from build123d import *

# Parameters (mm, degrees)
SKETCH1_R           = 13
BOSS_EXTRUDE1_DEPTH = 25
SKETCH2_R           = 4
CUT_EXTRUDE1_DEPTH  = 8
SKETCH4_W           = 4.368412871
SKETCH4_H           = 18.958156908


with BuildPart() as part:
    # Sketch1 → Boss-Extrude1 (new body)
    with BuildSketch(Plane(origin=(0, 0, 0), x_dir=(1, 0, 0), z_dir=(0, 1, 0))):
        with Locations(Location((0, 0, 0), (0, 0, 270))):
            Circle(SKETCH1_R)
    extrude(amount=BOSS_EXTRUDE1_DEPTH)

    # Sketch2 → Cut-Extrude1 (cut)
    with BuildSketch(Plane(origin=(0, 25, 0), x_dir=(1, 0, 0), z_dir=(0, 1, 0))):
        with Locations(Location((0, 0, 0), (0, 0, 270))):
            Circle(SKETCH2_R)
    extrude(amount=-CUT_EXTRUDE1_DEPTH, mode=Mode.SUBTRACT)

    # Sketch4 → Cut-Revolve1 (revolve, cut)
    with BuildSketch(Plane.XY, mode=Mode.PRIVATE) as cut_revolve1_sk:
        with BuildLine():
            ThreePointArc((0, 0), (-9.192388155, 3.807611845), (-13, 13))
            Line((-13, 13), (-13, -5.958156908))
            Line((-13, -5.958156908), (0, -5.958156908))
            Line((0, -5.958156908), (0, 0))
        make_face()
        with Locations((-15.184206436, 3.520921546)):
            Rectangle(SKETCH4_W, SKETCH4_H)
    revolve(cut_revolve1_sk.sketch.rotate(Axis((0, -5.958156908, 0), (0, 1, 0)), 270), axis=Axis((0, -5.958156908, 0), (0, 1, 0)), mode=Mode.SUBTRACT)


solid = part.part
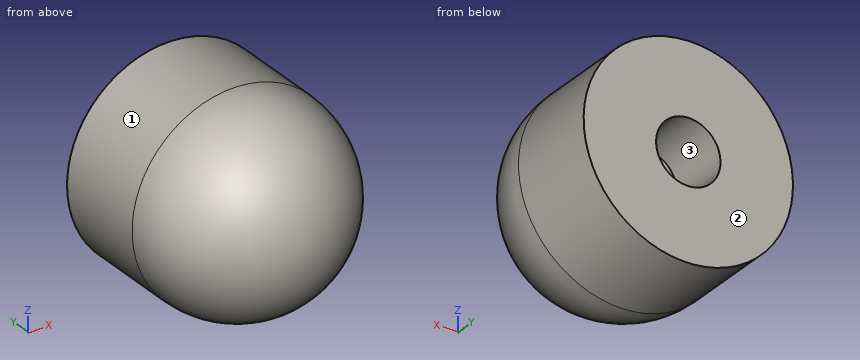
Source: CAD feature listing. Evaluate the final solid. Frame: model axes, mm. Face numbers are marked on the shaded views. Round coordinates to 2 decimals unless told otherwise and drop trailing zeros. Loops run counter-clockwise (first coordinate to the right, second up) from the corner with the lowest first, then second, coordinate; pieces in that order, holes last.
Q1. Section A-A, the plane y = 19.75. Return loops of the section in (x, z), plus the area to 3 significant figures.
Q2. Section B-B, the plane x = 0. Return loops of the section in (y, z).
Q3. Mould query, pull axis X, two halves, no side actions, for the marked faces 1, 2 and 3. Classes: pulls with the +X half, pulls with the -X half, needs draft (parallel to the pull), parting line crosses it, or undercut.
Q4. Section C-C, the plane z = 0. Return loops of the section in (x, y).
Q5. Section D-D, the plane y = 11. Return loops of the section in (x, z).
Q6. Ray query, line 1 (X direction, y = 22.5, z = 0); line 2 (Z direction, x = -5.25, y = 14); line 3 (X direction, y = 6.5, z = 4.5). Return the intervals inside material, ascending.
Q7. First-contact query: P1, Ø8, axis at x = -6.5, y = 17.5, coming from the +Z side; P2, Ø1.5, axis at x = -6.5, z = -9.5, coming from the -Y side; P3, Ø2, axis at x = -7, y = 2.5, coming from the -Z side. Flat tips, straight axial feed; report the tip coordinate or a pass-through.
Solutions:
1. outline: circle Ø26 at (0, 0); hole circle Ø8 at (0, 0)
1. area: 481 mm2
2. outline: (13, -13) - (25, -13) - (25, -4) - (17, -4) - (17, 4) - (25, 4) - (25, 13) - (13, 13) arc R13 ccw to start
3. face 1: parting line crosses it
3. face 2: needs draft
3. face 3: undercut
4. outline: (-13, 13) arc R13 ccw to (13, 13) - (13, 25) - (4, 25) - (4, 17) - (-4, 17) - (-4, 25) - (-13, 25) - close
5. outline: circle Ø25.69 at (0, 0)
6. line 1: x = -13 to -4, 4 to 13
6. line 2: z = -11.89 to 11.89
6. line 3: x = -10.32 to 10.32
7. P1: stops at z = 12.76
7. P2: stops at y = 5.71
7. P3: stops at z = -5.83
